```python
from build123d import *

# Parameters (mm, degrees)
SKIZZE1_W                       = 45
SKIZZE1_H                       = 65
AUFSATZ_LINEAR_AUSTRAGEN1_DEPTH = 2
SKIZZE3_W                       = 35
SKIZZE3_H                       = 42
SCHNITT_LINEAR_AUSTRAGEN1_DEPTH = 2
SKIZZE4_W                       = 2
SKIZZE4_H                       = 3
AUFSATZ_LINEAR_AUSTRAGEN2_DEPTH = 2
SKIZZE5_W                       = 2
SKIZZE5_H                       = 3
AUFSATZ_LINEAR_AUSTRAGEN3_DEPTH = 2
SKIZZE6_R                       = 1.6
SCHNITT_LINEAR_AUSTRAGEN2_DEPTH = 2


with BuildPart() as part:
    # Skizze1 → Aufsatz-Linear austragen1 (new body)
    with BuildSketch(Plane.XY):
        with Locations((22.5, 32.5)):
            Rectangle(SKIZZE1_W, SKIZZE1_H)
    extrude(amount=AUFSATZ_LINEAR_AUSTRAGEN1_DEPTH)

    # Skizze3 → Schnitt-Linear austragen1 (cut)
    with BuildSketch(Plane.XY.offset(2)):
        with Locations((22.5, 32.5)):
            Rectangle(SKIZZE3_W, SKIZZE3_H)
    extrude(amount=-SCHNITT_LINEAR_AUSTRAGEN1_DEPTH, mode=Mode.SUBTRACT)

    # Skizze4 → Aufsatz-Linear austragen2 (add)
    with BuildSketch(Plane(origin=(5, 0, 0), x_dir=(0, 0, -1), z_dir=(1, 0, 0))):
        with Locations((-1, 50.5)):
            Rectangle(SKIZZE4_W, SKIZZE4_H)
        with Locations((-1, 46)):
            Rectangle(SKIZZE4_W, SKIZZE4_H)
        with Locations((-1, 41.5)):
            Rectangle(SKIZZE4_W, SKIZZE4_H)
        with Locations((-1, 37)):
            Rectangle(SKIZZE4_W, SKIZZE4_H)
        with Locations((-1, 32.5)):
            Rectangle(SKIZZE4_W, SKIZZE4_H)
        with Locations((-1, 28)):
            Rectangle(SKIZZE4_W, SKIZZE4_H)
        with Locations((-1, 23.5)):
            Rectangle(SKIZZE4_W, SKIZZE4_H)
        with Locations((-1, 19)):
            Rectangle(SKIZZE4_W, SKIZZE4_H)
        with Locations((-1, 14.5)):
            Rectangle(SKIZZE4_W, SKIZZE4_H)
    extrude(amount=AUFSATZ_LINEAR_AUSTRAGEN2_DEPTH)

    # Skizze5 → Aufsatz-Linear austragen3 (add)
    with BuildSketch(Plane.ZY.offset(-40)):
        with Locations((1, 50.5)):
            Rectangle(SKIZZE5_W, SKIZZE5_H)
        with Locations((1, 46)):
            Rectangle(SKIZZE5_W, SKIZZE5_H)
        with Locations((1, 41.5)):
            Rectangle(SKIZZE5_W, SKIZZE5_H)
        with Locations((1, 37)):
            Rectangle(SKIZZE5_W, SKIZZE5_H)
        with Locations((1, 32.5)):
            Rectangle(SKIZZE5_W, SKIZZE5_H)
        with Locations((1, 28)):
            Rectangle(SKIZZE5_W, SKIZZE5_H)
        with Locations((1, 23.5)):
            Rectangle(SKIZZE5_W, SKIZZE5_H)
        with Locations((1, 19)):
            Rectangle(SKIZZE5_W, SKIZZE5_H)
        with Locations((1, 14.5)):
            Rectangle(SKIZZE5_W, SKIZZE5_H)
    extrude(amount=AUFSATZ_LINEAR_AUSTRAGEN3_DEPTH)

    # Skizze6 → Schnitt-Linear austragen2 (cut)
    with BuildSketch(Plane.XY.offset(2)):
        with Locations((7, 58)):
            Circle(SKIZZE6_R)
        with Locations((38, 58)):
            Circle(SKIZZE6_R)
        with Locations((38, 7)):
            Circle(SKIZZE6_R)
        with Locations((7, 7)):
            Circle(SKIZZE6_R)
    extrude(amount=-SCHNITT_LINEAR_AUSTRAGEN2_DEPTH, mode=Mode.SUBTRACT)


solid = part.part
```
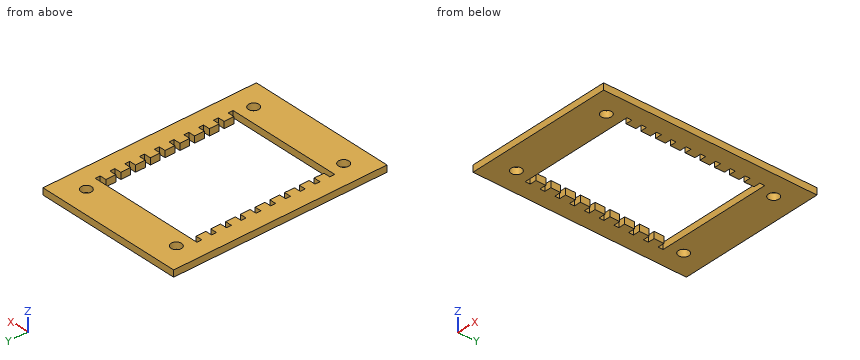
Geometry check sheet. Reference: the model listing, model coordinates, mm. Give positions to 0.01 mm unless a question says otherwise; leave off trailing zeros. Order: outer loops, then holes, each group sorted by start corner. A loop starts at its lowest first (then second) coordinate and runs counter-clockwise, first axis right, second up.
1. Section check A-A, the plane y = 7. Enter the section's corners in (x, z), and give its area (3 significant figures).
2. Gauge pin test, flat end, axial feed: pin 1 Ø1.9 at (x, y) = (7, 58) entering from -Z. Record the tip position at first contact, or that the pin passes through.
3. Section check B-B, the plane x = 31. Enter the section's corners in (y, z).
4. Section check C-C, the plane y = 36.5. Enter the section's corners in (x, z).
5. Thickness scan on L1, parallel to Y at x = 21.5, z = 0.35; L2, parallel to X at y = 21, z = 0.25; L3, parallel to X at y = 24, z = 0.45. Record the ranges inside material, lowest first.
6. Section check D-D, the plane z = 0.8. Give the number of separate pieces and of enclosed holes in the cut face, and give its area (3 significant figures).
Values follow:
1. outline: (0, 0) - (5.4, 0) - (5.4, 2) - (0, 2) - close; (8.6, 0) - (36.4, 0) - (36.4, 2) - (8.6, 2) - close; (39.6, 0) - (45, 0) - (45, 2) - (39.6, 2) - close
1. area: 77.2 mm2
2. pin 1: passes through
3. outline: (0, 0) - (11.5, 0) - (11.5, 2) - (0, 2) - close; (53.5, 0) - (65, 0) - (65, 2) - (53.5, 2) - close
4. outline: (0, 0) - (7, 0) - (7, 2) - (0, 2) - close; (38, 0) - (45, 0) - (45, 2) - (38, 2) - close
5. L1: y = 0 to 11.5, 53.5 to 65
5. L2: x = 0 to 5, 40 to 45
5. L3: x = 0 to 7, 38 to 45
6. separate pieces: 1
6. enclosed holes: 5
6. area: 1,530 mm2
